from build123d import *
from build123d.topology import SkipClean

# Parameters (mm, degrees)
BOSS_EXTRUDE1_DEPTH     = 20
SKETCH2_W               = 60
SKETCH2_H               = 12
BOSS_EXTRUDE2_DEPTH     = 5
SKETCH3_R               = 4
BOSS_EXTRUDE3_DEPTH     = 10
CUT_EXTRUDE1_DEPTH      = 38.939846984
CUT_EXTRUDE1_DEPTH_BACK = 38.939846984
SKETCH3_3_R             = 4


with BuildPart() as part:
    # Sketch1 → Boss-Extrude1 (new body)
    with BuildSketch(Plane(origin=(0, 0, 0), x_dir=(1, 0, 0), z_dir=(0, 1, 0))):
        Polygon((20.061919505, 0.724458204), (29.349845201, 0.724458204), (29.349845201, 12.724458204), (-30.650154799, 12.724458204), (-30.650154799, 0.724458204), (-21.176470588, 0.724458204), (-21.176470588, 5.851393189), (20.061919505, 5.851393189), align=None)
    extrude(amount=BOSS_EXTRUDE1_DEPTH)

    # Sketch2 → Boss-Extrude2 (add)
    with BuildSketch(Plane.XZ):
        with Locations((-0.650154799, -6.724458204)):
            Rectangle(SKETCH2_W, SKETCH2_H)
    extrude(amount=-BOSS_EXTRUDE2_DEPTH)

    # Sketch3 → Boss-Extrude3 (add)
    with BuildSketch(Plane.XY.offset(-5.851393189)):
        with BuildLine():
            Line((-8, 6), (-8, -11.858632677))
            ThreePointArc((-8, -11.858632677), (0, -19.858632677), (8, -11.858632677))
            Line((8, -11.858632677), (8, 6))
            ThreePointArc((8, 6), (0, 14), (-8, 6))
        make_face()
        with Locations(Location((0, 6, 0), (0, 0, 194.477512186))):
            Circle(SKETCH3_R, mode=Mode.SUBTRACT)
    extrude(amount=BOSS_EXTRUDE3_DEPTH)

    # Sketch3_3 → Cut-Extrude1 (cut, two sides: drawn at the far end of the back side and taken through both)
    with SkipClean():  # the faces are left unmerged after this step: merging them gives an invalid solid
        with BuildSketch(Plane.XY.offset(-5.851393189).offset(-CUT_EXTRUDE1_DEPTH_BACK)):
            with Locations((0, 6)):
                Circle(SKETCH3_3_R)
        extrude(amount=CUT_EXTRUDE1_DEPTH + CUT_EXTRUDE1_DEPTH_BACK, mode=Mode.SUBTRACT)


solid = part.part
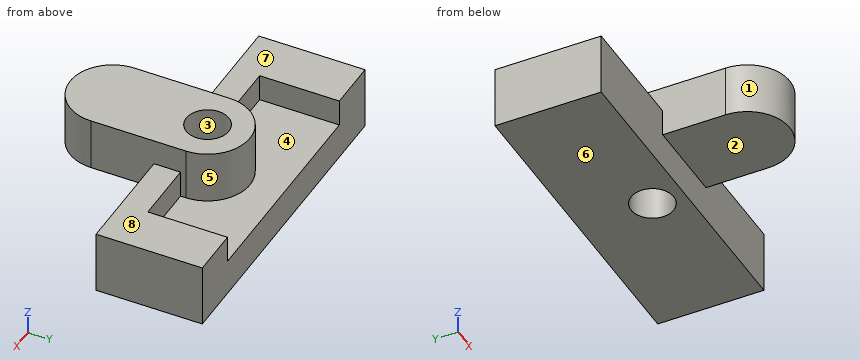
Verification items for the finished model (mm, model axes). Face numbers are marked on the shaded views. A direction names the side the tool comes from. Give positions to 0.01 mm unless a question says otherwise; leave off trailing zeros. Loops run counter-clockwise (first coordinate to the right, second up) from the corner with the lowest first, then second, coordinate; pieces in that order, holes last.
1) Set-up check for the marked faces 5, 6, 7 and 8: record each of +Z, -Z, +X, -X, +Y, -Y from which the full face is reachable in a straight line by a thin tool's end or side.
2) Sectioned sample at C-C, the plane z = -11.25. Enter the section's corners in (x, y).
3) Sectioned sample at B-B, the plane y = 16. Enter the section's corners in (x, z), then the cut area to 3 significant figures.
4) Thickness scan on line 1 along Y through (x, z) = (0, -1); line 2 along X through (y, z) = (6, -8.5); line 3 along Y through (x, z) = (0, -6). Record the ranges inside material, lowest first.
5) Draft check along X on the marked faces 1, 2, 3 and 4. Enter one of: pulls with the +X half, pulls with the -X half, needs draft (parallel to the pull), parting line crosses it, or undercut.
6) Sectioned sample at A-A, the plane x = 0. Enter the section's corners in (y, z), then the cut area to 3 significant figures.
7) Sectioned sample at D-D, the plane y = 4. Enter the section's corners in (x, z), then the cut area to 3 significant figures.
8) Depth check by flat-ended pin: pin 1 Ø6 at (x, y) = (-21, 5.5) entering from +Z; pin 2 Ø4 at (y, z) = (-13, -1.5) entering from -X; pin 3 Ø6 at (x, z) = (-12, -6.5) entering from -Y. Enter the tip coordinate at first touch or a pass-through.
Answers:
1. face 5: +Z, +Y
1. face 6: -Z, +X, -X, +Y, -Y
1. face 7: +Z, -X, +Y, -Y
1. face 8: +Z, +X, +Y, -Y
2. outline: (-30.65, 0) - (29.35, 0) - (29.35, 20) - (-30.65, 20) - close; hole circle Ø8 at (0, 6)
3. outline: (-30.65, -12.72) - (29.35, -12.72) - (29.35, -0.72) - (20.06, -0.72) - (20.06, -5.85) - (-21.18, -5.85) - (-21.18, -0.72) - (-30.65, -0.72) - close
3. area: 509 mm2
4. line 1: y = -19.86 to 2, 10 to 14
4. line 2: x = -30.65 to -4, 4 to 29.35
4. line 3: y = 0 to 2, 10 to 20
5. face 1: parting line crosses it
5. face 2: needs draft
5. face 3: undercut
5. face 4: undercut
6. outline: (-19.86, -5.85) - (0, -5.85) - (0, -12.72) - (2, -12.72) - (2, 4.15) - (-19.86, 4.15) - close; (10, -12.72) - (20, -12.72) - (20, -5.85) - (14, -5.85) - (14, 4.15) - (10, 4.15) - close
6. area: 341 mm2
7. outline: (-30.65, -12.72) - (-3.46, -12.72) - (-3.46, 4.15) - (-8, 4.15) - (-8, -0.72) - (-30.65, -0.72) - close; (3.46, -12.72) - (29.35, -12.72) - (29.35, -0.72) - (8, -0.72) - (8, 4.15) - (3.46, 4.15) - close
7. area: 681 mm2
8. pin 1: stops at z = -0.72
8. pin 2: stops at x = -8
8. pin 3: stops at y = 0
